```python
from build123d import *

# Parameters (mm, degrees)
LPATTERN1_COUNT     = 3
LPATTERN1_PITCH     = 88.9
LPATTERN1_2_COUNT   = 4
LPATTERN1_2_PITCH   = 88.9
SKETCH3_R           = 38.1
BOSS_EXTRUDE1_DEPTH = 1.27


with BuildPart() as part:
    # Sketch1 → Revolve1 (revolve)
    with BuildSketch(Plane.YZ, mode=Mode.PRIVATE) as revolve1_sk:
        Polygon((38.1, 0), (31.381942035, -38.1), (0, -38.1), (0, -39.37), (32.447598567, -39.37), (39.165656532, -1.27), (44.45, -1.27), (44.45, 0), align=None)
    revolve(revolve1_sk.sketch.rotate(Axis((0, 0, -38.1), (0, 0, 1)), 90), axis=Axis((0, 0, -38.1), (0, 0, 1)))


with BuildPart() as lpattern1_1:
    # LPattern1: pattern copy
    add(part.part.moved(Location(Vector(0, -1, 0) * (1 * LPATTERN1_PITCH))))


with BuildPart() as lpattern1_2:
    # LPattern1: pattern copy
    add(part.part.moved(Location(Vector(0, -1, 0) * (2 * LPATTERN1_PITCH))))


with BuildPart() as lpattern1_2_1:
    # LPattern1 2: pattern copy
    add(part.part.moved(Location(Vector(1, 0, 0) * (1 * LPATTERN1_2_PITCH))))


with BuildPart() as lpattern1_2_2:
    # LPattern1 2: pattern copy
    add(part.part.moved(Location(Vector(1, 0, 0) * (2 * LPATTERN1_2_PITCH))))


with BuildPart() as lpattern1_2_3:
    # LPattern1 2: pattern copy
    add(part.part.moved(Location(Vector(1, 0, 0) * (3 * LPATTERN1_2_PITCH))))


with BuildPart() as lpattern1_2_4:
    # LPattern1 2: pattern copy
    add(lpattern1_1.part.moved(Location(Vector(1, 0, 0) * (1 * LPATTERN1_2_PITCH))))


with BuildPart() as lpattern1_2_5:
    # LPattern1 2: pattern copy
    add(lpattern1_1.part.moved(Location(Vector(1, 0, 0) * (2 * LPATTERN1_2_PITCH))))


with BuildPart() as lpattern1_2_6:
    # LPattern1 2: pattern copy
    add(lpattern1_1.part.moved(Location(Vector(1, 0, 0) * (3 * LPATTERN1_2_PITCH))))


with BuildPart() as lpattern1_2_7:
    # LPattern1 2: pattern copy
    add(lpattern1_2.part.moved(Location(Vector(1, 0, 0) * (1 * LPATTERN1_2_PITCH))))


with BuildPart() as lpattern1_2_8:
    # LPattern1 2: pattern copy
    add(lpattern1_2.part.moved(Location(Vector(1, 0, 0) * (2 * LPATTERN1_2_PITCH))))


with BuildPart() as lpattern1_2_9:
    # LPattern1 2: pattern copy
    add(lpattern1_2.part.moved(Location(Vector(1, 0, 0) * (3 * LPATTERN1_2_PITCH))))


with BuildPart() as part_1:
    add(part.part)

    add(lpattern1_1.part)  # Boss-Extrude1 merges LPattern1_1

    add(lpattern1_2.part)  # Boss-Extrude1 merges LPattern1_2

    add(lpattern1_2_1.part)  # Boss-Extrude1 merges LPattern1 2_1

    add(lpattern1_2_2.part)  # Boss-Extrude1 merges LPattern1 2_2

    add(lpattern1_2_3.part)  # Boss-Extrude1 merges LPattern1 2_3

    add(lpattern1_2_4.part)  # Boss-Extrude1 merges LPattern1 2_4

    add(lpattern1_2_5.part)  # Boss-Extrude1 merges LPattern1 2_5

    add(lpattern1_2_6.part)  # Boss-Extrude1 merges LPattern1 2_6

    add(lpattern1_2_7.part)  # Boss-Extrude1 merges LPattern1 2_7

    add(lpattern1_2_8.part)  # Boss-Extrude1 merges LPattern1 2_8

    add(lpattern1_2_9.part)  # Boss-Extrude1 merges LPattern1 2_9
    # Sketch3 → Boss-Extrude1 (add)
    with BuildSketch(Plane.XY):
        with BuildLine():
            ThreePointArc((44.45, -177.8), (31.430896424, -209.230896424), (0, -222.25))
            Line((0, -222.25), (266.7, -222.25))
            ThreePointArc((266.7, -222.25), (235.269103576, -146.369103576), (311.15, -177.8))
            Line((311.15, -177.8), (311.15, 0))
            ThreePointArc((311.15, 0), (235.269103576, -31.430896424), (266.7, 44.45))
            Line((266.7, 44.45), (0, 44.45))
            ThreePointArc((0, 44.45), (31.430896424, 31.430896424), (44.45, 0))
            ThreePointArc((44.45, 0), (0, -44.45), (-44.45, 0))
            Line((-44.45, 0), (-44.45, -177.8))
            ThreePointArc((-44.45, -177.8), (0, -133.35), (44.45, -177.8))
        make_face()
        with Locations((88.9, -177.8)):
            Circle(SKETCH3_R, mode=Mode.SUBTRACT)
        with Locations((177.8, -177.8)):
            Circle(SKETCH3_R, mode=Mode.SUBTRACT)
        with Locations((0, -88.9)):
            Circle(SKETCH3_R, mode=Mode.SUBTRACT)
        with Locations((88.9, -88.9)):
            Circle(SKETCH3_R, mode=Mode.SUBTRACT)
        with Locations((88.9, 0)):
            Circle(SKETCH3_R, mode=Mode.SUBTRACT)
        with Locations((177.8, -88.9)):
            Circle(SKETCH3_R, mode=Mode.SUBTRACT)
        with Locations((266.7, -88.9)):
            Circle(SKETCH3_R, mode=Mode.SUBTRACT)
        with Locations((177.8, 0)):
            Circle(SKETCH3_R, mode=Mode.SUBTRACT)
    extrude(amount=-BOSS_EXTRUDE1_DEPTH)


solid = part_1.part
```
Geometry: final body of the model. Coordinates: model frame, mm. A direction names the side the tool comes from. Round coordinates to 2 decimals unless told otherwise and drop trailing zeros. Order: outer loops, then holes, each group sorted by start corner. A loop starts at its lowest first (then second) coordinate and runs counter-clockwise, first axis right, second up. Notation, with made-up numbers: M -29,26.5 L -23,26.5 A11 ccw -23,35.5 Z; hole C 40,-39 d8. An arc over 180 degrees is marked long. Use one line per item in the form item = value. Start each with the question number.
Q1. Access query for faces 1 (the face through (0, 0, -38.1)), 2 (the face through (133, -88, -1.27)), 3 (the face through (88, 0, -39.37)). Directions: +Z, -Z, +X, -X, +Y, -Y. A direction counts if a zero-diameter tool reaches every point of the face in a straight line with its end or side. Return the directions, or none.
Q2. Cut plane B-B (x = 88.9). Return loops of the section in (y, z).
Q3. Material intervals for line 1 (Y direction, x = 90, z = -14); line 2 (Y direction, x = 253.5, z = -20.5); line 3 (Z direction, x = 71.5, y = -113.5), sorted ascending. Write a range as [from, to].
Q4. Pin query (flat end, axial travel): pin 1 Ø19 at (x, y) = (267, -101) entering from +Z; pin 2 Ø12 at (x, z) = (155.5, -31.5) entering from +Y; pin 3 Ø8 at (x, y) = (203, -37) entering from -Z; pin 4 Ø2 at (x, y) = (48.5, -188.5) entering from +Z. Return the tip coordinate at first contact, or that it passes through.
Q5. Mould query, pull axis Y, two halves, no side actions, for faces 4 (the face through (267, 0, -38.1)), 5 (the face through (0, 0, -39.37)), 6 (the face through (297.783, -209.575, -0.626)). Classes: +Y half, -Y half, draft (parallel to the pull), parting line (faces both ways), or undercut.
Q6. Cut plane A-A (z = -28). Count the separate pieces of the cut face and the enclosed holes in it, and give its area (3 significant figures).
Geometry results:
q1.face_1 = +Z
q1.face_2 = -Z
q1.face_3 = -Z, +X, -X, +Y, -Y
q2.outline = M -222.25,-1.27 L -216.97,-1.27 L -210.25,-39.37 L -145.35,-39.37 L -138.63,-1.27 L -128.07,-1.27 L -121.35,-39.37 L -56.45,-39.37 L -49.73,-1.27 L -39.17,-1.27 L -32.45,-39.37 L 32.45,-39.37 L 39.17,-1.27 L 44.45,-1.27 L 44.45,0 L 38.1,0 L 31.38,-38.1 L -31.38,-38.1 L -38.1,0 L -50.8,0 L -57.52,-38.1 L -120.28,-38.1 L -127,0 L -139.7,0 L -146.42,-38.1 L -209.18,-38.1 L -215.9,0 L -222.25,0 Z
q3.line_1 = [-214.7, -213.41], [-142.19, -140.9], [-125.8, -124.51], [-53.29, -52], [-36.9, -35.61], [35.61, 36.9]
q3.line_2 = [-211.05, -209.66], [-145.94, -144.55], [-122.15, -120.76], [-57.04, -55.65], [-33.25, -31.86], [31.86, 33.25]
q3.line_3 = [-39.37, -38.1]
q4.pin_1 = -38.1
q4.pin_2 = 29.86
q4.pin_3 = -1.27
q4.pin_4 = 0
q5.face_4 = undercut
q5.face_5 = draft
q5.face_6 = -Y half
q6.separate_pieces = 12
q6.enclosed_holes = 12
q6.area = 3,290 mm^2
